Geometry: final body of the model. Coordinates: model frame, mm. Face numbers are marked on the shaded views. A direction names the side the tool comes from. Give positions to 0.01 mm unless a question says otherwise; leave off trailing zeros. Order: outer loops, then holes, each group sorted by start corner. A loop starts at its lowest first (then second) coordinate and runs counter-clockwise, first axis right, second up. Notation, with made-up numbers: (72, -2) - (126, -2) arc R19 ccw to (126, 9) - close; hole circle Ø9 at (46, -27.75). An arc over 180 degrees is marked (long way). One line per item, written item: value.
```python
from build123d import *

# Parameters (mm, degrees)
SKETCH5_W           = 25
SKETCH5_H           = 50
BOSS_EXTRUDE2_DEPTH = 135
SKETCH6_W           = 20
SKETCH6_H           = 45
CUT_EXTRUDE1_DEPTH  = 135
SKETCH7_R           = 4
CUT_EXTRUDE4_DEPTH  = 13.5


with BuildPart() as part:
    # Sketch5 → Boss-Extrude2 (new body)
    with BuildSketch(Plane(origin=(0, 0, 0), x_dir=(0, 0, -1), z_dir=(1, 0, 0))):
        Rectangle(SKETCH5_W, SKETCH5_H)
    extrude(amount=-BOSS_EXTRUDE2_DEPTH)

    # Sketch6 → Cut-Extrude1 (cut)
    with BuildSketch(Plane(origin=(0, 0, 0), x_dir=(0, 0, -1), z_dir=(1, 0, 0))):
        Rectangle(SKETCH6_W, SKETCH6_H)
    extrude(amount=-CUT_EXTRUDE1_DEPTH, mode=Mode.SUBTRACT)

    # Sketch7 → Cut-Extrude4 (cut, through all)
    with BuildSketch(Plane.XY):
        with Locations((-57.600290454, 3.389089755)):
            Circle(SKETCH7_R)
    extrude(amount=CUT_EXTRUDE4_DEPTH, mode=Mode.SUBTRACT)


solid = part.part
```
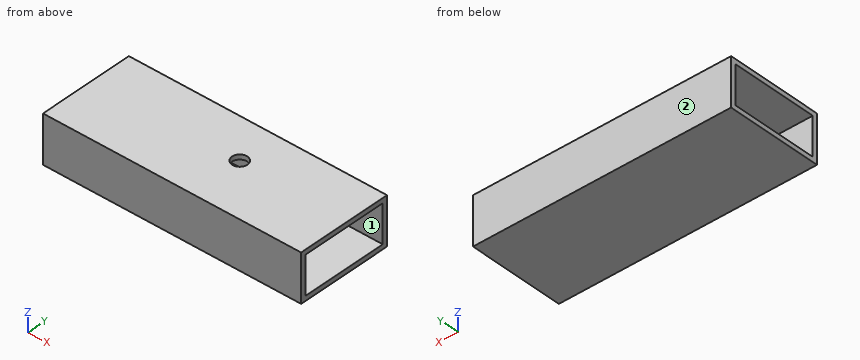
1) Section A-A, the plane y = -12. Return loops of the section in (x, z), then the cut area to 3 significant figures.
Answers below:
outline: (-135, -12.5) - (0, -12.5) - (0, -10) - (-135, -10) - close; (-135, 10) - (0, 10) - (0, 12.5) - (-135, 12.5) - close
area: 675 mm^2
2) Section C-C, the plane x = -12. Return loops of the section in (y, z).
Answers below:
outline: (-25, -12.5) - (25, -12.5) - (25, 12.5) - (-25, 12.5) - close; hole (-22.5, -10) - (22.5, -10) - (22.5, 10) - (-22.5, 10) - close
3) First-contact query: pin 1 (7 mm diameter, centred on x = -57.6, y = 3.39, fed in from +Z). Flat tip, straight axial feed; report the tip coordinate or a pass-through.
Answers below:
pin 1: z = -10
4) Section B-B, the plane z = -3. Return loops of the section in (x, y), then the cut area to 3 significant figures.
Answers below:
outline: (-135, -25) - (0, -25) - (0, -22.5) - (-135, -22.5) - close; (-135, 22.5) - (0, 22.5) - (0, 25) - (-135, 25) - close
area: 675 mm^2
5) Material intervals for line 1 along Z through (x, y) = (-41, 7); line 2 along Y through (x, z) = (-117.5, 4.75), sorted ascending.
Answers below:
line 1: -12.5 to -10, 10 to 12.5
line 2: -25 to -22.5, 22.5 to 25
6) Set-up query: the marked faces 1 and 2. Return all of +Z, -Z, +X, -X, +Y, -Y with unobstructed straight access to the full face (end or side cutting, diameter ignored); none if empty.
Answers below:
face 1: +X, -X
face 2: +Z, -Z, +X, -X, +Y
